Design review of the part built by this model. Coordinates are the model's own, in mm. A direction names the side the tool comes from. Give positions to 0.01 mm unless a question says otherwise; leave off trailing zeros. Write each loop counter-clockwise with the first axis right and the second up, starting at its lowest first coordinate (ties: lowest second). Pieces come first, ordered by that corner, then holes. Notation, with made-up numbers: (40.25, 16) - (57.25, 16) arc R7 cw to (57.25, 27) - close; hole circle Ø8 at (12.5, -5.5). An arc over 180 degrees is marked (long way). Write each question's results on one line, items separated by ' | '. Start each with the question number.
from build123d import *

# Parameters (mm, degrees)
BOSS_EXTRUDE1_DEPTH = 12


with BuildPart() as part:
    # Sketch1 → Boss-Extrude1 (new body)
    with BuildSketch(Plane(origin=(0, 0, 0), x_dir=(0, 0, -1), z_dir=(1, 0, 0))):
        Polygon((0, 5.773502692), (-5, 2.886751346), (-5, -2.886751346), (0, -5.773502692), (5, -2.886751346), (5, 2.886751346), align=None)
    extrude(amount=-BOSS_EXTRUDE1_DEPTH)

    # Sketch2 → Cut-Revolve4 (revolve, cut)
    with BuildSketch(Plane.XY, mode=Mode.PRIVATE) as cut_revolve4_sk:
        Polygon((0, 5), (-0.446581987, 5.773502692), (0, 5.773502692), align=None)
        with BuildLine():
            Line((-4.409080445, 5.773502692), (-13.863248654, 5.773502692))
            Line((-13.863248654, 5.773502692), (-13.863248654, 0))
            Line((-13.863248654, 0), (-12, 0))
            ThreePointArc((-12, 0), (-10.608757211, 3.358757211), (-7.25, 4.75))
            Line((-7.25, 4.75), (-5, 4.75))
            Line((-5, 4.75), (-4.409080445, 5.773502692))
        make_face()
        Polygon((-10.136751346, 0), (-8.693375673, 2.5), (0, 2.5), (0, 0), align=None)
    revolve(cut_revolve4_sk.sketch.rotate(Axis((-12, 0, 0), (1, 0, 0)), 180), axis=Axis((-12, 0, 0), (1, 0, 0)), mode=Mode.SUBTRACT)


solid = part.part
Q1. Insertion check: P1, Ø1.5, axis at x = -1.5, z = -2, coming from the -Y side; P2, Ø6, axis at x = -10, z = 0, coming from the -Y side; P3, Ø2, axis at x = -3.5, z = -3.5, coming from the +Y side. Each pin has a flat end and moves straight along its axis. Give the tip position at first contact, or say it passes through.
Q2. Add section B-B on x = -6.5. State the section outline as (y, z) points.
Q3. For line 1 along Z through (x, y) = (-4.25, 0); line 2 along Y through (x, z) = (-0.5, 1); line 3 along X through (y, z) = (-2.5, 0.5), list the stretches that pass through material, from the lowest coordinate up. Write a range as [from, to].
Q4. Add section A-A on x = -2.25. State the section outline as (y, z) points.
Q5. Machinability: for faces 4 (the face through (-4.3, 2.5, -0.1)), 5 (the face through (-2, 0, -5)), 6 (the face through (-6.109, 1.03, 4.637)), which of the approach directions +Z, -Z, +X, -X, +Y, -Y give a long, thin tool a straight path to every point of the face, cutting with its end or side? Answer none if there is none.
Q6. The part is to be moulded in two halves that separate along Y. For faces 1 (the face through (-0.11, -2.58, 4.5)), 2 (the face through (-2.394, 4.31, -2.535)), 3 (the face through (-9.9, 0.1, 0.4)), say which applies: +Y half, -Y half, draft (parallel to the pull), parting line (faces both ways), or undercut.
Result:
1) P1: stops at y = -5.05 | P2: stops at y = -4.75 | P3: stops at y = 4.33
2) outline: circle Ø9.5 at (0, 0); hole circle Ø5 at (0, 0)
3) line 1: z = [-5, -2.5], [2.5, 5] | line 2: y = [-5.2, -2.29], [2.29, 5.2] | line 3: x = [-11.26, 0]
4) outline: (-5.77, 0) - (-2.89, -5) - (2.89, -5) - (5.77, 0) - (2.89, 5) - (-2.89, 5) - close; hole circle Ø5 at (0, 0)
5) face 4: +X | face 5: -Z, +X, -X, +Y, -Y | face 6: -X
6) face 1: -Y half | face 2: +Y half | face 3: undercut
